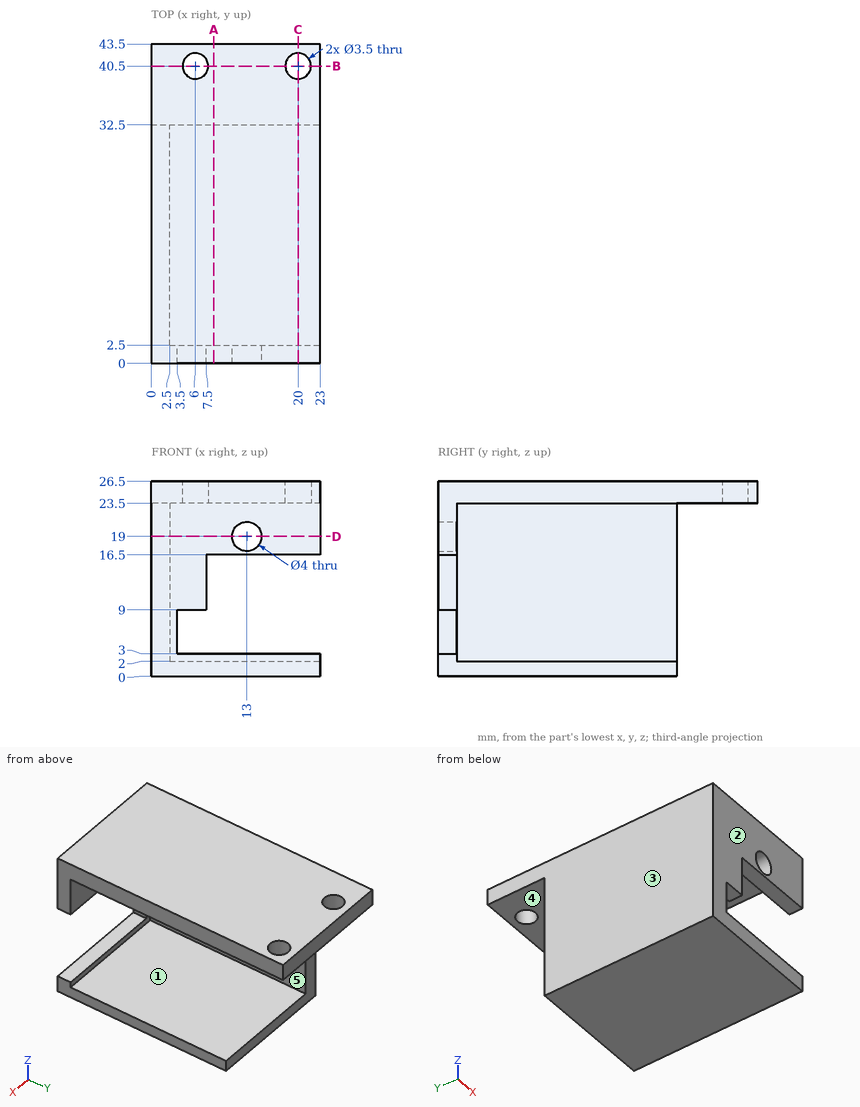
Part print with two shaded views. Sizes in mm from the minimum x, y, z corner. A direction names the side the tool comes from. Round coordinates to 2 decimals unless told otherwise and drop trailing zeros. Write each loop counter-clockwise with the first axis right and the second up, starting at its lowest first coordinate (ties: lowest second). Pieces come first, ordered by that corner, then holes. Notation, with made-up numbers: (43.5, 84) -> (48.5, 84) arc R33 cw to (48.5, 114) -> close; hole circle Ø1 at (47, -35). An arc over 180 degrees is marked (long way). Put each result on its own line as item: value.
Item 1: Tool access for the marked faces 1 and 2: list every direction of +Z, -Z, +X, -X, +Y, -Y with a clear straight run to the whole face (end or side of a thin tool).
Here are the results:
face 1: +X, +Y
face 2: +Z, -Z, +X, -X, -Y
Item 2: Flat gauge pins, fed straight in: P1, Ø5.5, axis at x = 6, y = 40.5, coming from the -Z side; P2, Ø0.8, axis at y = 1, z = 6, coming from the +X side; P3, Ø8, axis at y = 7, z = 16.5, coming from the +X side. Where does each tip first touch, or does it go through?
Here are the results:
P1: stops at z = 23.5
P2: stops at x = 3.5
P3: stops at x = 2.5
Item 3: Two-plate mould, pull along X, no slides. Class the marked faces 3, 4 and 5: pulls with the +X half, pulls with the -X half, needs draft (parallel to the pull), parting line crosses it, or undercut.
Here are the results:
face 3: pulls with the -X half
face 4: needs draft
face 5: pulls with the +X half
Item 4: Slice it at B-B, the plane y = 40.5. Give the cut face in (x, z), plus the area to 3 significant figures.
Here are the results:
outline: (0, 23.5) -> (4.25, 23.5) -> (4.25, 26.5) -> (0, 26.5) -> close; (7.75, 23.5) -> (18.25, 23.5) -> (18.25, 26.5) -> (7.75, 26.5) -> close; (21.75, 23.5) -> (23, 23.5) -> (23, 26.5) -> (21.75, 26.5) -> close
area: 48.0 mm^2
Item 5: Wall check: probe 1 along Z at (x, y) = (13, 1.15); probe 2 along Y at (x, z) = (20, 24.45); probe 3 along Z at (x, y) = (20, 24). Give the ranges that are in metal, low to high. Write a range as from..to.
Here are the results:
probe 1: z = 0..3, 16.5..17, 21..26.5
probe 2: y = 0..38.75, 42.25..43.5
probe 3: z = 0..2, 23.5..26.5
Item 6: Slice it at D-D, the plane z = 19. Give the cut face in (x, y), plus the area to 4 significant figures.
Here are the results:
outline: (0, 0) -> (11, 0) -> (11, 2.5) -> (2.5, 2.5) -> (2.5, 32.5) -> (0, 32.5) -> close; (15, 0) -> (23, 0) -> (23, 2.5) -> (15, 2.5) -> close
area: 122.5 mm^2
Item 7: Slice it at A-A, the plane x = 8.5. Give the cut face in (y, z).
Here are the results:
outline: (0, 0) -> (32.5, 0) -> (32.5, 2) -> (2.5, 2) -> (2.5, 3) -> (0, 3) -> close; (0, 16.5) -> (2.5, 16.5) -> (2.5, 23.5) -> (43.5, 23.5) -> (43.5, 26.5) -> (0, 26.5) -> close
Item 8: Slice it at C-C, the plane x = 20. Give the cut face in (y, z).
Here are the results:
outline: (0, 0) -> (32.5, 0) -> (32.5, 2) -> (2.5, 2) -> (2.5, 3) -> (0, 3) -> close; (0, 16.5) -> (2.5, 16.5) -> (2.5, 23.5) -> (38.75, 23.5) -> (38.75, 26.5) -> (0, 26.5) -> close; (42.25, 23.5) -> (43.5, 23.5) -> (43.5, 26.5) -> (42.25, 26.5) -> close
